```python
from build123d import *

# Parameters (mm, degrees)
CHAMFER_SIZE    = 1
SKETCH003_W     = 12
SKETCH003_H     = 50
POCKET001_DEPTH = 10.5


with BuildPart() as part:
    # Sketch002 → Revolution (revolve)
    with BuildSketch(Plane.XZ):
        Polygon((32.72376, 0), (32.72376, -24), (29.72376, -24), (29.72376, -17.5), (31.22376, -16), (29.72376, -14.5), (29.72376, -3), (3.75, -3), (3.75, 0), align=None)
    revolve(axis=Axis((0, 0, 0), (0, 0, 1)))

    # Chamfer
    chamfer_edges = [part.edges().sort_by_distance(p)[0] for p in [
        (-32.72376, 0, 0),
    ]]
    chamfer(chamfer_edges, length=CHAMFER_SIZE)

    # Sketch003 (on Face6 of Chamfer) → Pocket001 (cut)
    with BuildSketch(Plane(origin=(0, 0, -24), x_dir=(1, 0, 0), z_dir=(0, 0, -1))):
        with Locations((0, -25)):
            Rectangle(SKETCH003_W, SKETCH003_H)
    extrude(amount=-POCKET001_DEPTH, mode=Mode.SUBTRACT)


solid = part.part
```
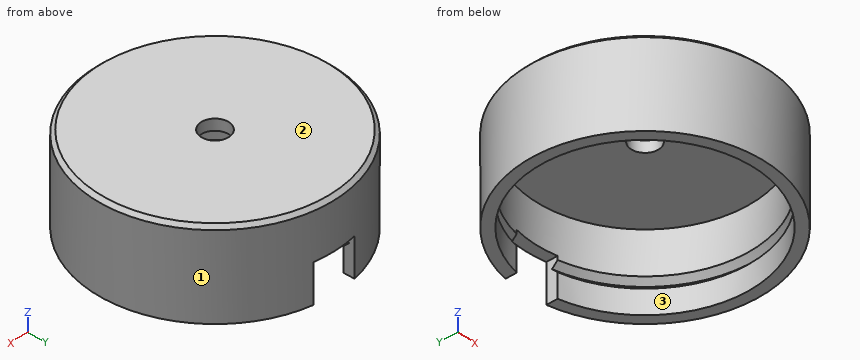
Source: CAD feature listing. Evaluate the final solid. Frame: model axes, mm. Face numbers are marked on the shaded views. Round coordinates to 2 decimals unless told otherwise and drop trailing zeros. Loops run counter-clockwise (first coordinate to the right, second up) from the corner with the lowest first, then second, coordinate; pieces in that order, holes last. Notation, with made-up numbers: M 43,47.25 L 71,47.25 A18 ccw 71,65.25 Z; hole C 12.25,-32.5 d4. An arc over 180 degrees is marked long. Use a Markdown table: item, result. Add a question column.
1. Line query: line 1 (Y direction, x = 0, z = -5.5); line 2 (Y direction, x = 0, z = -1.05); line 3 (Z direction, x = 22.5, y = 5). Output: solid intervals per line, ascending.
2. Section query B-B on y = 0. Return the cut outline in (x, z), then the cut area to 3 significant figures.
3. Section query A-A on x = 0. Return the cut outline in (y, z), then the cut area to 3 significant figures.
4. Mould query, pull axis Y, two halves, no side actions, for the marked faces 1, 2 and 3. Classes: pulls with the +Y half, pulls with the -Y half, needs draft (parallel to the pull), parting line crosses it, or undercut.
5. Contact query for flat-ended pins moving along their axis: P1, Ø4.5, axis at x = 0, y = 0, coming from the +Z side (1 decimal); P2, Ø4, axis at x = -1.5, y = 30, coming from the -Z side; P3, Ø4, axis at x = 4.5, z = -11, coming from the -Y side; P4, Ø2, axis at x = -17.5, z = -18.5, coming from the +Y side. Output: stop coordinate, or through.
Reported:
| question | item | result |
|---|---|---|
| 1 | line 1 | y = -32.72 to -29.72, 29.72 to 32.72 |
| 1 | line 2 | y = -32.72 to -3.75, 3.75 to 32.72 |
| 1 | line 3 | z = -3 to 0 |
| 2 | outline | M -32.72,-24 L -29.72,-24 L -29.72,-17.5 L -31.22,-16 L -29.72,-14.5 L -29.72,-3 L -3.75,-3 L -3.75,0 L -31.72,0 L -32.72,-1 Z; M 3.75,-3 L 29.72,-3 L 29.72,-14.5 L 31.22,-16 L 29.72,-17.5 L 29.72,-24 L 32.72,-24 L 32.72,-1 L 31.72,0 L 3.75,0 Z |
| 2 | area | 294 mm² |
| 3 | outline | M -32.72,-24 L -29.72,-24 L -29.72,-17.5 L -31.22,-16 L -29.72,-14.5 L -29.72,-3 L -3.75,-3 L -3.75,0 L -31.72,0 L -32.72,-1 Z; M 3.75,-3 L 29.72,-3 L 29.72,-13.5 L 32.72,-13.5 L 32.72,-1 L 31.72,0 L 3.75,0 Z |
| 3 | area | 265 mm² |
| 4 | face 1 | parting line crosses it |
| 4 | face 2 | needs draft |
| 4 | face 3 | undercut |
| 5 | P1 | passes through |
| 5 | P2 | stops at z = -13.5 |
| 5 | P3 | stops at y = -32.63 |
| 5 | P4 | stops at y = 28.26 |
